Autodesk Inventor part; units mm, degrees
ref_plane "YZ Plane" through (0, 0, 0) normal (1, 0, 0) x (0, 1, 0)
ref_plane "XZ Plane" through (0, 0, 0) normal (0, 1, 0) x (-1, 0, 0)
ref_plane "XY Plane" through (0, 0, 0) normal (0, 0, 1) x (1, 0, 0)
sketch "Sketch1" plane through (0, 0, 0) normal (0, 0, 1) x (1, 0, 0)
  line L0 (5, 0) -> (115.5, 0)
  line L1 (115.5, 0) -> (115.5, 64)
  line L2 (115.5, 64) -> (0, 64)
  line L3 (0, 64) -> (0, 5)
  line L4 (0, 5) -> (5, 0)
  line L5 (33.5, 37.5) -> (64.5, 37.5) construction
  line L6 (64.5, 37.5) -> (64.5, 6.5) construction
  line L7 (64.5, 6.5) -> (33.5, 6.5) construction
  line L8 (33.5, 6.5) -> (33.5, 37.5) construction
  line L9 (27.62, 43.38) -> (70.38, 43.38) construction
  line L10 (70.38, 43.38) -> (70.38, 0.62) construction
  line L11 (70.38, 0.62) -> (27.62, 0.62) construction
  line L12 (27.62, 0.62) -> (27.62, 43.38) construction
  circle A0 centre (33.5, 6.5) radius 1.6
  circle A1 centre (64.5, 6.5) radius 1.6
  circle A2 centre (64.5, 37.5) radius 1.6
  circle A3 centre (33.5, 37.5) radius 1.6
  circle A4 centre (49, 22) radius 11.5
  circle A5 centre (26, 22) radius 4
  point P0 (0, 0)
  point P1 (49, 37.5)
  point P2 (64.5, 22)
  point P3 (70.38, 22)
  point P4 (49, 43.38)
  dimension "d0" = 45
  dimension "d1" = 31
  dimension "d2" = 42.76
  dimension "d3" = 3.2
  dimension "d4" = 23
  dimension "d5" = 8
  dimension "d6" = 23
  dimension "d8" = 115.5
  dimension "d9" = 42
  dimension "d10" = 5
  dimension "d11" = 22
  dimension "d63" = 26
extrude "Extrusion1" add sketch "Sketch1" along normal blind 6.5
sketch "Sketch3" plane through (0, 0, 6.5) normal (0, 0, 1) x (1, 0, 0)
  circle A0 centre (26, 22) radius 4
  circle A1 centre (64.5, 37.5) radius 1.6
  line L0 (5, 0) -> (115.5, 0)
  circle A2 centre (20, 6) radius 2.25
  circle A3 centre (93.75, 49.5) radius 2.25
  line L1 (115.5, 0) -> (115.5, 64)
  point P0 (0, 0)
  dimension "d29" = 4.5
  dimension "d30" = 6
  dimension "d31" = 6
  dimension "d32" = 12
  dimension "d64" = 21.75
extrude "Extrusion3" cut sketch "Sketch3" against normal through all contours A2 | A3
sketch "Sketch4" plane through (0, 0, 6.5) normal (0, 0, 1) x (1, 0, 0)
  line L0 (115.5, 0) -> (115.5, 64)
  line L1 (0, 64) -> (0, 5)
  line L2 (5, 0) -> (115.5, 0)
  line L3 (3, 22) -> (9.5, 22)
  line L4 (9.5, 22) -> (9.5, 14)
  line L5 (9.5, 14) -> (3, 14)
  line L6 (3, 14) -> (3, 22)
  line L7 (3, 45) -> (9.5, 45)
  line L8 (9.5, 45) -> (9.5, 37)
  line L9 (9.5, 37) -> (3, 37)
  line L10 (3, 37) -> (3, 45)
  line L11 (106, 45) -> (112.5, 45)
  line L12 (112.5, 45) -> (112.5, 37)
  line L13 (112.5, 37) -> (106, 37)
  line L14 (106, 37) -> (106, 45)
  line L15 (106, 22) -> (112.5, 22)
  line L16 (112.5, 22) -> (112.5, 14)
  line L17 (112.5, 14) -> (106, 14)
  line L18 (106, 14) -> (106, 22)
  line L19 (3, 37) -> (9.5, 22) construction
  line L20 (3, 22) -> (9.5, 37) construction
  line L21 (106, 37) -> (112.5, 22) construction
  line L22 (106, 22) -> (112.5, 37) construction
  circle A0 centre (6.25, 29.5) radius 2.25
  circle A1 centre (109.25, 29.5) radius 2.25
  point P0 (0, 0)
  dimension "d36" = 6.5
  dimension "d37" = 8
  dimension "d38" = 8
  dimension "d39" = 6.5
  dimension "d40" = 15
  dimension "d41" = 3
  dimension "d42" = 3
  dimension "d43" = 14
  dimension "d44" = 4.5
extrude "Extrusion4" cut sketch "Sketch4" against normal through all
sketch "Sketch5" plane through (0, 0, 6.5) normal (0, 0, 1) x (1, 0, 0)
  line L0 (115.5, 64) -> (0, 64)
  line L1 (0, 64) -> (0, 5)
  line L2 (17.75, 64) -> (22.25, 64)
  line L3 (22.25, 47.7) -> (17.75, 47.7)
  line L4 (24.75, 59) -> (24.75, 51.7)
  line L5 (15.25, 51.7) -> (15.25, 59)
  line L6 (17.75, 47.7) -> (17.75, 51.7)
  line L7 (17.75, 59) -> (17.75, 64)
  line L8 (22.25, 64) -> (22.25, 59)
  line L9 (22.25, 51.7) -> (22.25, 47.7)
  line L10 (15.25, 59) -> (17.75, 59)
  line L11 (22.25, 59) -> (24.75, 59)
  line L12 (24.75, 51.7) -> (22.25, 51.7)
  line L13 (17.75, 51.7) -> (15.25, 51.7)
  line L14 (72.75, 64) -> (77.25, 64)
  line L15 (77.25, 47.7) -> (72.75, 47.7)
  line L16 (79.75, 59) -> (79.75, 51.7)
  line L17 (70.25, 51.7) -> (70.25, 59)
  line L18 (72.75, 47.7) -> (72.75, 51.7)
  line L19 (72.75, 59) -> (72.75, 64)
  line L20 (77.25, 64) -> (77.25, 59)
  line L21 (77.25, 51.7) -> (77.25, 47.7)
  line L22 (70.25, 59) -> (72.75, 59)
  line L23 (77.25, 59) -> (79.75, 59)
  line L24 (79.75, 51.7) -> (77.25, 51.7)
  line L25 (72.75, 51.7) -> (70.25, 51.7)
  point P0 (0, 0)
  point P1 (20, 47.7)
  point P2 (75, 47.7)
  dimension "d47" = 4.5
  dimension "d48" = 2.5
  dimension "d49" = 2.5
  dimension "d50" = 5
  dimension "d51" = 7.3
  dimension "d52" = 4
  dimension "d53" = 4.5
  dimension "d54" = 2.5
  dimension "d55" = 2.5
  dimension "d56" = 5
  dimension "d57" = 7.3
  dimension "d58" = 4
  dimension "d59" = 20
  dimension "d60" = 55
extrude "Extrusion5" cut sketch "Sketch5" against normal through all
chamfer "Chamfer1" distance 2 angle 45 1 edges at (115.5, 0, 3.25)
sketch "Sketch6" plane through (0, 0, 6.5) normal (0, 0, 1) x (1, 0, 0)
  line L0 (72.75, 64) -> (22.25, 64)
  line L1 (47.5, 59.3812) -> (43.5, 61.6906)
  line L2 (43.5, 61.6906) -> (43.5, 64)
  line L3 (51.5, 64) -> (51.5, 61.6906)
  line L4 (51.5, 61.6906) -> (47.5, 59.3812)
  line L5 (43.5, 64) -> (51.5, 64)
  point P0 (0, 0)
  point P1 (47.5, 64)
  dimension "d68" = 8
extrude "Extrusion6" cut sketch "Sketch6" against normal through all
equation "\"d39\" = d36"
properties part number "z_motor_mount" material "Plywood, Finish"
Read the model definition and answer for the solid it produces. Units are mm, in the model's axes. A direction names the side the tool comes from. Round coordinates to 2 decimals unless told otherwise and drop trailing zeros. Write each loop counter-clockwise with the first axis right and the second up, starting at its lowest first coordinate (ties: lowest second). Pieces come first, ordered by that corner, then holes. Notation, with made-up numbers: (26, 23.5) - (80, 23.5) arc R29 cw to (80, 59.5) - close; hole circle Ø1 at (59, 58.25). An arc over 180 degrees is marked (long way). One line per question, with ' | ' between items. Start each with the question number.
1. Each of these flat-tipped pins is pushed along its axis until it touches: pin 1 (3 mm diameter, centred on x = 49, z = 2.5, fed in from +Y); pin 2 (2.5 mm diameter, centred on x = 20, y = 6, fed in from -Z); pin 3 (2 mm diameter, centred on x = 20.5, z = 3.5, fed in from +Y). Where does it stop, or does it pass through?
2. For faces 4 (the face through (58, 0, 3)), 5 (the face through (6, 14, 3)), 6 (the face through (45.53, 60.52, 3.3)), determine the directions among +Z, -Z, +X, -X, +Y, -Y from which every point of the face is accessible in a straight line to the end or side of a thin tool.
3. Find the intervals of material crossed by probe 1 along Y at (x, z) = (33.5, 2.5); probe 2 along X at (y, z) = (23.5, 4.75); probe 3 along X at (y, z) = (7.5, 3.5), in increasing order. Write a range as [from, to].
4. Section A-A (x = 26) is taken. Determine the outline of the cut face in (y, z), and give its area (3 significant figures).
5. Section C-C (y = 29.5) is taken. Determine the outline of the cut face in (x, z), and give its area (3 significant figures).
6. Section D-D (x = 64.5) is taken. Determine the outline of the cut face in (y, z).
7. Section B-B (x = 6.25) is taken. Determine the outline of the cut face in (y, z), and give its area (3 significant figures).
8. For a pull along X with two mould halves and no side action, classify faces 1 (the face through (23, 59, 3)), 2 (the face through (9, 64, 3)), 3 (the face through (3, 41, 3)) as +X half, -X half, draft (parallel to the pull), parting line (faces both ways), or undercut.
Filled in:
1) pin 1: y = 61.11 | pin 2: through | pin 3: y = 47.7
2) face 4: +Z, -Z, +X, -X, -Y | face 5: +Z, -Z | face 6: +Z, -Z, +Y
3) probe 1: [0, 4.9], [8.1, 35.9], [39.1, 64] | probe 2: [0, 22.29], [29.71, 37.6], [60.4, 115.5] | probe 3: [0, 18.32], [21.68, 32.25], [34.75, 63.25], [65.75, 115.5]
4) outline: (0, 0) - (18, 0) - (18, 6.5) - (0, 6.5) - close; (26, 0) - (64, 0) - (64, 6.5) - (26, 6.5) - close | area: 364 mm²
5) outline: (0, 0) - (4, 0) - (4, 6.5) - (0, 6.5) - close; (8.5, 0) - (40.28, 0) - (40.28, 6.5) - (8.5, 6.5) - close; (57.72, 0) - (107, 0) - (107, 6.5) - (57.72, 6.5) - close; (111.5, 0) - (115.5, 0) - (115.5, 6.5) - (111.5, 6.5) - close | area: 579 mm²
6) outline: (0, 0) - (4.9, 0) - (4.9, 6.5) - (0, 6.5) - close; (8.1, 0) - (35.9, 0) - (35.9, 6.5) - (8.1, 6.5) - close; (39.1, 0) - (64, 0) - (64, 6.5) - (39.1, 6.5) - close
7) outline: (0, 0) - (14, 0) - (14, 6.5) - (0, 6.5) - close; (22, 0) - (27.25, 0) - (27.25, 6.5) - (22, 6.5) - close; (31.75, 0) - (37, 0) - (37, 6.5) - (31.75, 6.5) - close; (45, 0) - (64, 0) - (64, 6.5) - (45, 6.5) - close | area: 283 mm²
8) face 1: undercut | face 2: draft | face 3: undercut
